from build123d import *

# Parameters (mm, degrees)
SKETCH_1_R          = 2.5
EXTRUDE_1_DEPTH     = 150
CUT_EXTRUDE_1_DEPTH = 153.242379078


with BuildPart() as part:
    # 草图1 → 凸台-拉伸1 (new body)
    with BuildSketch(Plane.XY):
        with BuildLine():
            Line((-25.95624704, -9.765592916), (-27.75624704, -9.765592916))
            Line((-27.75624704, -9.765592916), (-27.75624704, -15.165592916))
            ThreePointArc((-27.75624704, -15.165592916), (-27.316907212, -16.226253087), (-26.25624704, -16.665592916))
            Line((-26.25624704, -16.665592916), (-20.85624704, -16.665592916))
            Line((-20.85624704, -16.665592916), (-20.85624704, -14.865592916))
            Line((-20.85624704, -14.865592916), (-23.25624704, -14.865592916))
            Line((-23.25624704, -14.865592916), (-23.25624704, -13.062643071))
            Line((-23.25624704, -13.062643071), (-19.959196885, -9.765592916))
            Line((-19.959196885, -9.765592916), (-15.553297195, -9.765592916))
            Line((-15.553297195, -9.765592916), (-12.25624704, -13.062643071))
            Line((-12.25624704, -13.062643071), (-12.25624704, -14.865592916))
            Line((-12.25624704, -14.865592916), (-14.65624704, -14.865592916))
            Line((-14.65624704, -14.865592916), (-14.65624704, -16.665592916))
            Line((-14.65624704, -16.665592916), (-9.25624704, -16.665592916))
            ThreePointArc((-9.25624704, -16.665592916), (-8.195586868, -16.226253087), (-7.75624704, -15.165592916))
            Line((-7.75624704, -15.165592916), (-7.75624704, -9.765592916))
            Line((-7.75624704, -9.765592916), (-9.55624704, -9.765592916))
            Line((-9.55624704, -9.765592916), (-9.55624704, -12.165592916))
            Line((-9.55624704, -12.165592916), (-11.359196885, -12.165592916))
            Line((-11.359196885, -12.165592916), (-14.70212002, -8.822669781))
            Line((-14.70212002, -8.822669781), (-14.70212002, -4.50851605))
            Line((-14.70212002, -4.50851605), (-11.359196885, -1.165592916))
            Line((-11.359196885, -1.165592916), (-9.55624704, -1.165592916))
            Line((-9.55624704, -1.165592916), (-9.55624704, -3.565592916))
            Line((-9.55624704, -3.565592916), (-7.75624704, -3.565592916))
            Line((-7.75624704, -3.565592916), (-7.75624704, 1.834407084))
            ThreePointArc((-7.75624704, 1.834407084), (-8.195586868, 2.895067256), (-9.25624704, 3.334407084))
            Line((-9.25624704, 3.334407084), (-14.65624704, 3.334407084))
            Line((-14.65624704, 3.334407084), (-14.65624704, 1.534407084))
            Line((-14.65624704, 1.534407084), (-12.25624704, 1.534407084))
            Line((-12.25624704, 1.534407084), (-12.25624704, -0.26854276))
            Line((-12.25624704, -0.26854276), (-15.553297195, -3.565592916))
            Line((-15.553297195, -3.565592916), (-19.959196885, -3.565592916))
            Line((-19.959196885, -3.565592916), (-23.25624704, -0.26854276))
            Line((-23.25624704, -0.26854276), (-23.25624704, 1.534407084))
            Line((-23.25624704, 1.534407084), (-20.85624704, 1.534407084))
            Line((-20.85624704, 1.534407084), (-20.85624704, 3.334407084))
            Line((-20.85624704, 3.334407084), (-26.25624704, 3.334407084))
            ThreePointArc((-26.25624704, 3.334407084), (-27.316907212, 2.895067256), (-27.75624704, 1.834407084))
            Line((-27.75624704, 1.834407084), (-27.75624704, -3.565592916))
            Line((-27.75624704, -3.565592916), (-25.95624704, -3.565592916))
            Line((-25.95624704, -3.565592916), (-25.95624704, -1.165592916))
            Line((-25.95624704, -1.165592916), (-24.153297195, -1.165592916))
            Line((-24.153297195, -1.165592916), (-20.81037406, -4.50851605))
            Line((-20.81037406, -4.50851605), (-20.81037406, -8.822669781))
            Line((-20.81037406, -8.822669781), (-24.153297195, -12.165592916))
            Line((-24.153297195, -12.165592916), (-25.95624704, -12.165592916))
            Line((-25.95624704, -12.165592916), (-25.95624704, -9.765592916))
        make_face()
        with Locations((-17.75624704, -6.665592916)):
            Circle(SKETCH_1_R, mode=Mode.SUBTRACT)
    extrude(amount=EXTRUDE_1_DEPTH)

    # 草图2 → 切除-拉伸1 (cut, through all)
    with BuildSketch(Plane.ZY.offset(27.75624704)):
        Polygon((0, -16.665592916), (20, 3.334407084), (0, 3.334407084), align=None)
        Polygon((150, -16.665592916), (130, 3.334407084), (150, 3.334407084), align=None)
    extrude(amount=-CUT_EXTRUDE_1_DEPTH, mode=Mode.SUBTRACT)


solid = part.part
Read the model definition and answer for the solid it produces. Units are mm, in the model's axes. A direction names the side the tool comes from. Round coordinates to 2 decimals unless told otherwise and drop trailing zeros. Order: outer loops, then holes, each group sorted by start corner. A loop starts at its lowest first (then second) coordinate and runs counter-clockwise, first axis right, second up. Notation, with made-up numbers: (39.25, 42.25) - (93.25, 42.25) arc R24 cw to (93.25, 72.25) - close; hole circle Ø6 at (84, -35). An arc over 180 degrees is marked (long way). Use one line per item in the form item = value. Start each with the question number.
(1) For faces 5 (the face through (-22, 1.534, 74)), 6 (the face through (-18, -9.766, 74)), 7 (the face through (-20.81, -7, 74)), determine the directions among +Z, -Z, +X, -X, +Y, -Y from which every point of the face is accessible in a straight line to the end or side of a thin tool.
(2) Flat-ended cylindrical pins translate along their axes: pin 1 Ø6 at (x, y) = (-12, -2.5) entering from +Z; pin 2 Ø0.5 at (y, z) = (3, 48) entering from +X; pin 3 Ø12 at (x, y) = (-13, -4) entering from -Z. Find the tip coordinate at first contact, or state that the pin passes through.
(3) Determine the mould class of faces 1 (the face through (-9.556, -2, 74)), 2 (the face through (-20.118, -9.028, 7.638)), 3 (the face through (-21.631, -11.437, 74)), 4 (the face through (-27.756, -12, 74)) for opening direction X: +X half, -X half, draft (parallel to the pull), parting line (faces both ways), or undercut.
(4) The part is cut by section A-A (x = -18). Give the vertices of the cut face in (y, z).
(5) Find the intervals of material crossed by line 1 along Y through (x, z) = (-11, 57.5); line 2 along X through (y, z) = (2, 63); line 3 along X through (y, z) = (-14.75, 79), in increasing order. Write a range as from..to.
Checked values:
q1.face_5 = +Z, -Z
q1.face_6 = +Z, -Z, -Y
q1.face_7 = +Z, -Z, -X
q2.pin_1 = 137.58
q2.pin_2 = -8.07
q2.pin_3 = 6.69
q3.face_1 = undercut
q3.face_2 = draft
q3.face_3 = undercut
q3.face_4 = -X half
q4.outline = (-9.77, 6.9) - (-9.15, 7.51) - (-9.15, 142.49) - (-9.77, 143.1) - close; (-4.18, 12.49) - (-3.57, 13.1) - (-3.57, 136.9) - (-4.18, 137.51) - close
q5.line_1 = -16.67..-12.17, -1.17..3.33
q5.line_2 = -27.75..-20.86, -14.66..-7.77
q5.line_3 = -27.76..-23.26, -12.26..-7.76
